```python
from build123d import *

# Parameters (mm, degrees)
SKETCH_1_R      = 5
EXTRUDE_1_DEPTH = 52
SKETCH_2_R      = 4.5
EXTRUDE_2_DEPTH = 10
EXTRUDE_START   = 20
SKETCH_3_R      = 4.5
EXTRUDE_3_DEPTH = 20


with BuildPart() as part:
    # 草图1 → 凸台-拉伸1 (new, symmetric)
    with BuildSketch(Plane.XY):
        with Locations(Location((0, 0, 0), (0, 0, 180))):
            Circle(SKETCH_1_R)
    extrude(amount=EXTRUDE_1_DEPTH, both=True)

    # 草图2 → 凸台-拉伸2 (add)
    with BuildSketch(Plane(origin=(0, 0, -52), x_dir=(-1, 0, 0), z_dir=(0, 0, -1))):
        with Locations(Location((0, 0, 0), (0, 0, 180))):
            Circle(SKETCH_2_R)
    extrude(amount=EXTRUDE_2_DEPTH)

    # 草图3 → 凸台-拉伸3 (add)
    with BuildSketch(Plane.XY.offset(52).offset(EXTRUDE_START)):
        Circle(SKETCH_3_R)
    extrude(amount=-EXTRUDE_3_DEPTH)


solid = part.part
```
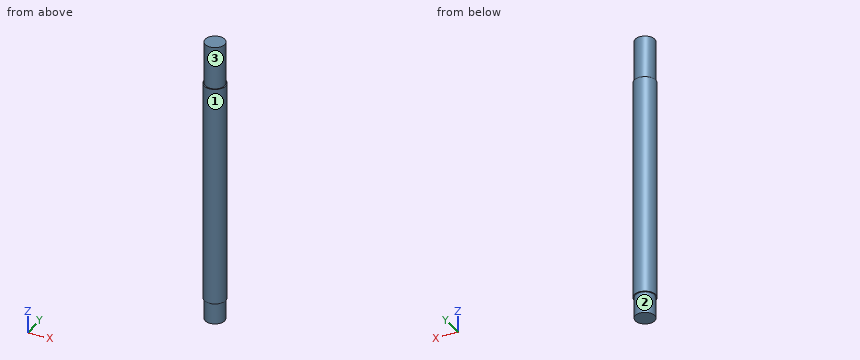
Part model, mm, in its own coordinate system. Face numbers are marked on the shaded views. A direction names the side the tool comes from. Coordinates: 2 decimals unless noted, no trailing zeros. Loops run counter-clockwise (first coordinate to the right, second up) from the corner with the lowest first, then second, coordinate; pieces in that order, holes last. Notation, with made-up numbers: (72, -29) - (77, -29) arc R14 ccw to (77, -24) - close; hole circle Ø7 at (-1.75, 73). An arc over 180 degrees is marked (long way). Write item = value, one per line. Start each with the question number.
Item 1: Cut at A-A, the plane y = 0. Give the cut face in (x, z), and give its area (3 significant figures).
Item 2: Wall check: L1, parallel to Y at x = 0.5, z = -22; L2, parallel to X at y = -2.25, z = -47; L3, parallel to Y at x = -4.5, z = -29.5. Give the ranges that are in metal, low to high. Write a range as from..to.
Item 3: Flat gauge pins, fed straight in: pin 1 Ø5 at (y, z) = (-2.5, -20.5) entering from +X; pin 2 Ø1.5 at (x, z) = (-2.5, 12) entering from -Y; pin 3 Ø1 at (x, z) = (2.5, 53.5) entering from +Y; pin 4 Ø1.5 at (x, z) = (-2, 20.5) entering from -Y. Where does each tip first touch, or does it go through?
Item 4: Cut at C-C, the plane z = 7. Give the cut face in (x, y), and give its area (3 significant figures).
Item 5: 3-axis set-ups, long thin cutter, end or side, ignore diameter. For the marked faces 1, 2 and 3: which of +Z, -Z, +X, -X, +Y, -Y reach the whole face in a straight line?
The answers:
q1.outline = (-5, -52) - (-4.5, -52) - (-4.5, -62) - (4.5, -62) - (4.5, -52) - (5, -52) - (5, 52) - (4.5, 52) - (4.5, 72) - (-4.5, 72) - (-4.5, 52) - (-5, 52) - close
q1.area = 1,310 mm2
q2.L1 = -4.97..4.97
q2.L2 = -4.47..4.47
q2.L3 = -2.18..2.18
q3.pin_1 = 5
q3.pin_2 = -4.68
q3.pin_3 = 4.03
q3.pin_4 = -4.84
q4.outline = circle Ø10 at (0, 0)
q4.area = 78.5 mm2
q5.face_1 = +Z, -Z
q5.face_2 = -Z
q5.face_3 = +Z
